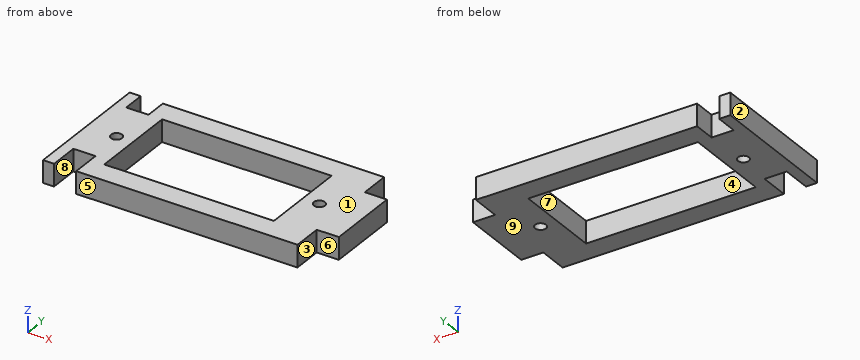
```python
from build123d import *

# Parameters (mm, degrees)
SKETCH_1_R      = 1.5
SKETCH_1_R_2    = 0.75
EXTRUDE_9_DEPTH = 3


with BuildPart() as part:
    # 草图1 → 凸台-拉伸9 (new body)
    # profile 1 of 2: a face of its own
    with BuildSketch(Plane.XY):
        Polygon((37.5, -4), (37.5, -14), (34.5, -14), (34.5, -18), (4.5, -18), (4.5, -14), (1.5, -14), (1.5, -18), (0, -18), (0, 0), (1.5, 0), (1.5, -3), (4.5, -3), (4.5, 0), (34.5, 0), (34.5, -4), align=None)
        with Locations((36, -9)):
            Circle(SKETCH_1_R, mode=Mode.SUBTRACT)
        with Locations((4.1, -9)):
            Circle(SKETCH_1_R_2, mode=Mode.SUBTRACT)
        with Locations((31.6, -9)):
            Circle(SKETCH_1_R_2, mode=Mode.SUBTRACT)
        Polygon((29.35, -15), (6.35, -15), (6.35, -9), (6.35, -3), (29.35, -3), align=None, mode=Mode.SUBTRACT)
    # profile 2 of 2: a face of its own
    with BuildSketch(Plane.XY):
        with Locations((36, -9)):
            Circle(SKETCH_1_R)
    extrude(amount=EXTRUDE_9_DEPTH)


solid = part.part
```
Verification items for the finished model (mm, model axes). Face numbers are marked on the shaded views. A direction names the side the tool comes from. Round coordinates to 2 decimals unless told otherwise and drop trailing zeros. Write each loop counter-clockwise with the first axis right and the second up, starting at its lowest first coordinate (ties: lowest second). Pieces come first, ordered by that corner, then holes. Notation, with made-up numbers: (49.5, 0) -> (92.5, 0) arc R14 ccw to (92.5, 14) -> close; hole circle Ø4 at (59, -12.75). An arc over 180 degrees is marked (long way). Write each question's results on one line, items separated by ' | '.
Q1. Go/stop test with flat-tipped pins: pin 1 Ø0.9 at (x, z) = (3, 1) entering from -Y; pin 2 Ø0.9 at (x, y) = (31.6, -9) entering from -Z; pin 3 Ø1.5 at (x, z) = (36.5, 2) entering from +Y; pin 4 Ø0.9 at (y, z) = (-16.5, 2) entering from +X. Record where each tip stops, or that it passes through.
Derived:
pin 1: stops at y = -14 | pin 2: passes through | pin 3: stops at y = -4 | pin 4: stops at x = 34.5
Q2. Sectioned sample at D-D, the plane z = 0.65. Record the boundary of the cut face in (x, y), and give its area (3 significant figures).
Derived:
outline: (0, -18) -> (1.5, -18) -> (1.5, -14) -> (4.5, -14) -> (4.5, -18) -> (34.5, -18) -> (34.5, -14) -> (37.5, -14) -> (37.5, -4) -> (34.5, -4) -> (34.5, 0) -> (4.5, 0) -> (4.5, -3) -> (1.5, -3) -> (1.5, 0) -> (0, 0) -> close; hole circle Ø1.5 at (4.1, -9); hole (6.35, -15) -> (29.35, -15) -> (29.35, -3) -> (6.35, -3) -> close; hole circle Ø1.5 at (31.6, -9) | area: 350 mm²
Q3. Sectioned sample at A-A, the plane x = 20. Record the boundary of the cut face in (y, z), and give its area (3 significant figures).
Derived:
outline: (-18, 0) -> (-15, 0) -> (-15, 3) -> (-18, 3) -> close; (-3, 0) -> (0, 0) -> (0, 3) -> (-3, 3) -> close | area: 18.0 mm²
Q4. Access from +Z, -Z, +X, -X, +Y, -Y to the whole of each face (thin tool, end or side, straight path). Record for the marked faces 5, 6, 7, 8 and 9.
Derived:
face 5: +Z, -Z, +X, -X, -Y | face 6: +Z, -Z, +X, -Y | face 7: +Z, -Z | face 8: +Z, -Z, -Y | face 9: -Z, +X, -X, +Y, -Y
Q5. Sectioned sample at B-B, the plane y = -15.5. Record the boundary of the cut face in (x, z).
Derived:
outline: (0, 0) -> (1.5, 0) -> (1.5, 3) -> (0, 3) -> close; (4.5, 0) -> (34.5, 0) -> (34.5, 3) -> (4.5, 3) -> close
Q6. Draft check along X on the marked faces 1, 2, 3 and 4. Enter one of: released by +X, released by -X, zero draft, split by the parting line, or undercut.
Derived:
face 1: zero draft | face 2: released by -X | face 3: released by +X | face 4: undercut
Q7. Thickness scan on probe 1 along Y at (x, z) = (22, 2.3); probe 2 along X at (y, z) = (-0.25, 2.35); probe 3 along X at (y, z) = (-13.75, 1.5). Record the ranges inside material, lowest first.
Derived:
probe 1: y = -18 to -15, -3 to 0 | probe 2: x = 0 to 1.5, 4.5 to 34.5 | probe 3: x = 0 to 6.35, 29.35 to 37.5
Q8. Sectioned sample at C-C, the plane y = -9. Record the boundary of the cut face in (x, z).
Derived:
outline: (0, 0) -> (3.35, 0) -> (3.35, 3) -> (0, 3) -> close; (4.85, 0) -> (6.35, 0) -> (6.35, 3) -> (4.85, 3) -> close; (29.35, 0) -> (30.85, 0) -> (30.85, 3) -> (29.35, 3) -> close; (32.35, 0) -> (37.5, 0) -> (37.5, 3) -> (32.35, 3) -> close
